from build123d import *

# Parameters (mm, degrees)
BOSS_EXTRUDE1_DEPTH = 3
FILLET2_R           = 2
CUT_EXTRUDE1_DEPTH  = 1


with BuildPart() as part:
    # Sketch1 → Boss-Extrude1 (new body)
    with BuildSketch(Plane(origin=(0, 0, 0), x_dir=(1, 0, 0), z_dir=(0, 1, 0))):
        with BuildLine():
            Line((9.261243058, 19.135372648), (-9.261243058, 19.135372648))
            Line((-9.261243058, 19.135372648), (-82.394201363, 9.715975022))
            ThreePointArc((-82.394201363, 9.715975022), (-86.756396558, 7.396125613), (-88.5, 2.773323949))
            Line((-88.5, 2.773323949), (-88.5, -5.301071921))
            ThreePointArc((-88.5, -5.301071921), (-86.876170995, -9.784015756), (-82.758061306, -12.187092669))
            Line((-82.758061306, -12.187092669), (0, -27.306813988))
            Line((0, -27.306813988), (82.758061306, -12.187092669))
            ThreePointArc((82.758061306, -12.187092669), (86.876170995, -9.784015756), (88.5, -5.301071921))
            Line((88.5, -5.301071921), (88.5, 2.773323949))
            ThreePointArc((88.5, 2.773323949), (86.756396558, 7.396125613), (82.394201363, 9.715975022))
            Line((82.394201363, 9.715975022), (9.261243058, 19.135372648))
        make_face()
    extrude(amount=BOSS_EXTRUDE1_DEPTH)

    # Fillet2
    fillet2_edges = [part.edges().sort_by_distance(p)[0] for p in [
        (0, 1.5, 27.306813988),
    ]]
    fillet(fillet2_edges, radius=FILLET2_R)

    # Sketch2 → Cut-Extrude1 (cut)
    with BuildSketch(Plane(origin=(0, 3, 0), x_dir=(1, 0, 0), z_dir=(0, 1, 0))):
        Polygon((-77.031853449, -13.233258633), (-75.158975168, -2.982026326), (-20.368957027, -12.9920458), (-22.241835309, -23.243278108), align=None)
        Polygon((20.368957027, -12.9920458), (22.241835309, -23.243278108), (77.031853449, -13.233258633), (75.158975168, -2.982026326), align=None)
    extrude(amount=-CUT_EXTRUDE1_DEPTH, mode=Mode.SUBTRACT)


solid = part.part
Verification items for the finished model (mm, model axes). Give positions to 0.01 mm unless a question says otherwise; leave off trailing zeros. Write each loop counter-clockwise with the first axis right and the second up, starting at its lowest first coordinate (ties: lowest second). Pieces come first, ordered by that corner, then holes.
(1) Cross-section at D-D (z = 7). Enter the section's corners in (x, y), plus the area to 3 significant figures.
(2) Cross-section at B-B (z = 18). Enter the section's corners in (x, y), plus the area to 3 significant figures.
(3) Material ranges on line 1 (Z direction, x = 52, y = 0.5); line 2 (Z direction, x = -46, y = 2.85); line 3 (X direction, y = 1.3, z = -4), recorded low to high.
(4) Mould release check, pull along X, two halves, no side actions. Record for faces 1 (the face through (48.147, 2.507, 7.917)), 2 (the face through (-42.136, 1.146, 19.609)), 3 (the face through (86.83, 1.48, 9.84)), 4 (the face through (-48, 2, 13)): +X half, -X half, draft (parallel to the pull), parting line (faces both ways), or undercut.
(5) Cross-section at C-C (x = 59). Enter the section's corners in (y, z), plus the area to 3 significant figures.
(6) Gauge pin test, flat end, axial feed: pin 1 (2 mm diameter, centred on x = 23.5, z = 19, fed in from +Y). Record the tip position at first contact, or that the pin passes through.
(7) Cross-section at A-A (y = 1.55). Enter the section's corners in (x, z), plus the area to 3 significant figures.
Worked out:
1. outline: (-88.29, 0) - (88.29, 0) - (88.29, 3) - (75.89, 3) - (75.89, 2) - (53.17, 2) - (53.17, 3) - (-53.17, 3) - (-53.17, 2) - (-75.89, 2) - (-75.89, 3) - (-88.29, 3) - close
1. area: 484 mm2
2. outline: (-50.94, 0) - (50.94, 0) - (50.94, 2) - (21.28, 2) - (21.28, 3) - (-21.28, 3) - (-21.28, 2) - (-50.94, 2) - close
2. area: 246 mm2
3. line 1: z = -13.63 to 17.81
3. line 2: z = -14.4 to 8.31
3. line 3: x = -88.39 to 88.39
4. face 1: undercut
4. face 2: -X half
4. face 3: +X half
4. face 4: undercut
5. outline: (0, -12.73) - (3, -12.73) - (3, 5.93) - (2, 5.93) - (2, 16.53) - (0, 16.53) - close
5. area: 77.2 mm2
6. pin 1: stops at y = 2
7. outline: (-88.5, -2.77) arc R7 ccw to (-82.39, -9.72) - (-9.26, -19.14) - (9.26, -19.14) - (82.39, -9.72) arc R7 ccw to (88.5, -2.77) - (88.5, 5.3) arc R7 ccw to (82.76, 12.19) - (0.36, 27.24) arc R2 ccw to (-0.36, 27.24) - (-82.76, 12.19) arc R7 ccw to (-88.5, 5.3) - close
7. area: 5,950 mm2
